Print and shaded views of the part. All mm, measured from the part's lowest x, y and z. A direction names the side the tool comes from. Round coordinates to 2 decimals unless told otherwise and drop trailing zeros. Write each loop counter-clockwise with the first axis right and the second up, starting at its lowest first coordinate (ties: lowest second). Pieces come first, ordered by that corner, then holes.
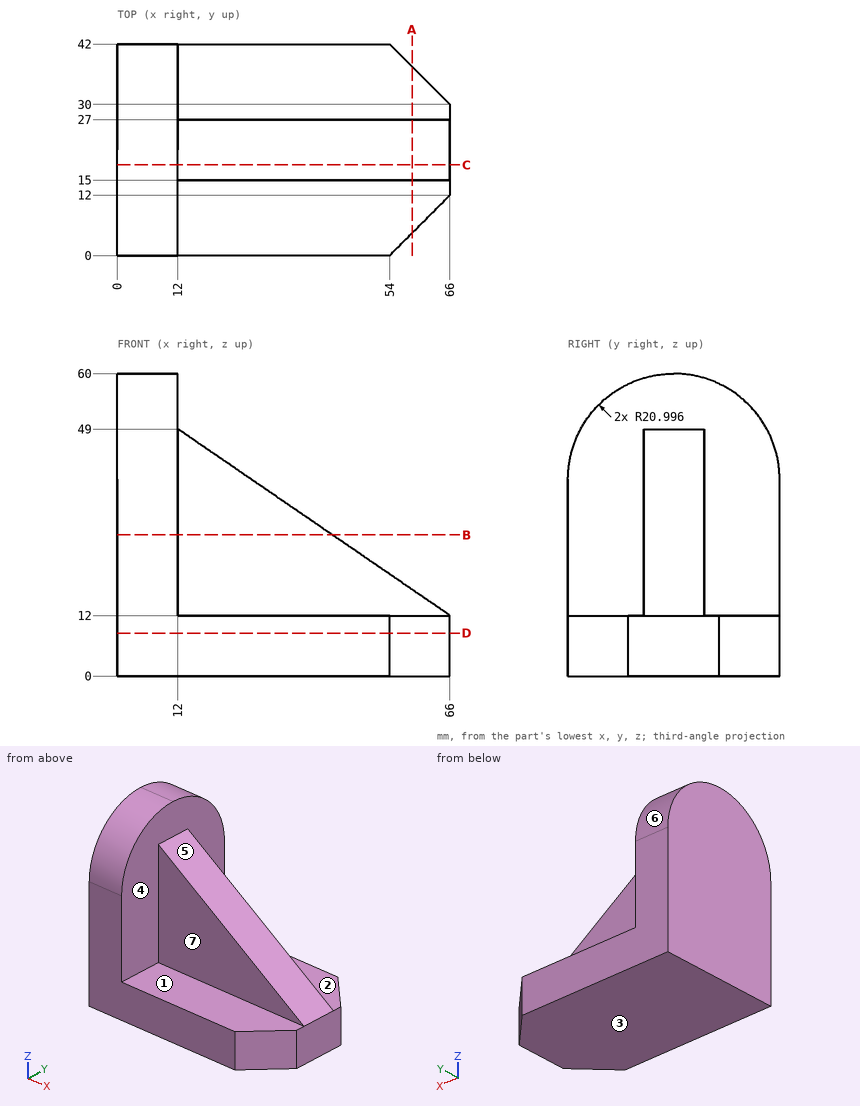
1) Slice it at D-D (z = 8.5). Write the cut outline in (x, y).
Results:
outline: (0, 0) - (54, 0) - (66, 12) - (66, 30) - (54, 42) - (0, 42) - close
2) Wall check: L1, parallel to X at y = 11, z = 39.5; L2, parallel to Y at x = 26, z = 17.5. Give the ranges that are in metal, low to high.
Results:
L1: x = 0 to 12
L2: y = 15 to 27
3) Mould opens along Y. For the marked faces 5, 6 and 7 say: released by +Y, released by -Y, zero draft, split by the parting line, or undercut.
Results:
face 5: zero draft
face 6: released by +Y
face 7: released by -Y
4) Slice it at B-B (z = 28). Write the cut outline in (x, y), plus the area to 3 significant figures.
Results:
outline: (0, 0) - (12, 0) - (12, 15) - (42.65, 15) - (42.65, 27) - (12, 27) - (12, 42) - (0, 42) - close
area: 872 mm2
5) Which spindle directions (+Z, -Z, +X, -X, +Y, -Y) get a long thin tool onto all of the face, cutting with end or side? Do the marked faces 1, 2, 3 and 4. Say none if no direction does.
Results:
face 1: +Z, +X, -Y
face 2: +Z, +X, +Y
face 3: -Z, +X, -X, +Y, -Y
face 4: +Z, +X
6) Slice it at A-A (x = 58.5). Write the cut outline in (y, z).
Results:
outline: (4.5, 0) - (37.5, 0) - (37.5, 12) - (27, 12) - (27, 17.14) - (15, 17.14) - (15, 12) - (4.5, 12) - close
7) Slice it at C-C (y = 18). Write the cut outline in (x, z) (1 decimal).
Results:
outline: (0, 0) - (66, 0) - (66, 12) - (12, 49) - (12, 59.8) - (0, 59.8) - close
8) Pin check, flat tips, straight feed: pin 1 Ø4.5 at (x, y) = (49, 5) entering from +Z; pin 2 Ø18.5 at (x, z) = (44, 30.5) entering from -Y; pin 3 Ø5 at (x, z) = (36, 34) entering from +Y. Stop position of each tip, or through.
Results:
pin 1: stops at z = 12
pin 2: stops at y = 15
pin 3: stops at y = 27
